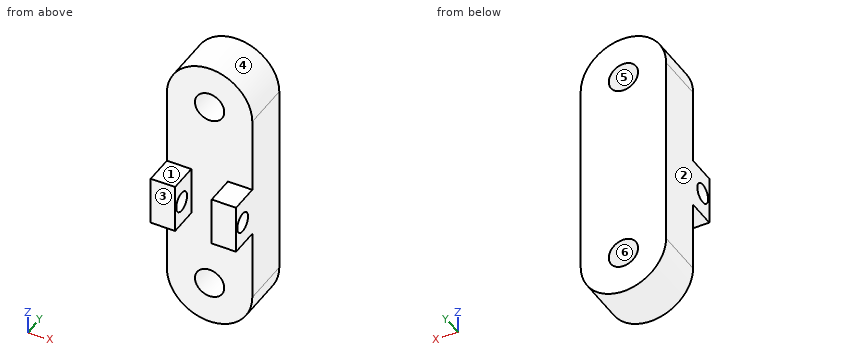
from build123d import *

# Parameters (mm, degrees)
SKETCH1_W             = 5
SKETCH1_H             = 10
BOSS_EXTRUDE1_DEPTH   = 6
BOSS_EXTRUDE1_2_DEPTH = 6
SKETCH2_R             = 2
CUT_EXTRUDE1_DEPTH    = 100
SKETCH4_R             = 3
BOSS_EXTRUDE2_DEPTH   = 10


with BuildPart() as part:
    # Sketch1 → Boss-Extrude1 (new body)
    with BuildSketch(Plane(origin=(0, 0, 0), x_dir=(1, 0, 0), z_dir=(0, 1, 0))):
        with Locations((-15, 5)):
            Rectangle(SKETCH1_W, SKETCH1_H)
    extrude(amount=BOSS_EXTRUDE1_DEPTH)


with BuildPart() as body_2:
    # Sketch1 → Boss-Extrude1 2 (new body)
    with BuildSketch(Plane(origin=(0, 0, 0), x_dir=(1, 0, 0), z_dir=(0, 1, 0))):
        with Locations((-2.5, 5)):
            Rectangle(SKETCH1_W, SKETCH1_H)
    extrude(amount=BOSS_EXTRUDE1_2_DEPTH)


with BuildPart() as cut_extrude1_tool:
    # Sketch2 → Cut-Extrude1 (new body)
    with BuildSketch(Plane(origin=(0, 0, 0), x_dir=(0, 0, -1), z_dir=(1, 0, 0))):
        with Locations((5, 2.43)):
            Circle(SKETCH2_R)
    extrude(amount=-CUT_EXTRUDE1_DEPTH)


with BuildPart() as part_1:
    add(part.part)

    # Cut-Extrude1: cut by cut_extrude1_tool
    add(cut_extrude1_tool.part, mode=Mode.SUBTRACT)



with BuildPart() as body_2_1:
    add(body_2.part)

    # Cut-Extrude1: cut by cut_extrude1_tool
    add(cut_extrude1_tool.part, mode=Mode.SUBTRACT)


with BuildPart() as part_2:
    add(part_1.part)

    add(body_2_1.part)  # Boss-Extrude2 merges body 2
    # Sketch4 → Boss-Extrude2 (add)
    with BuildSketch(Plane(origin=(0, 6, 0), x_dir=(1, 0, 0), z_dir=(0, 1, 0))):
        with BuildLine():
            Line((-17.5, -15.5), (-17.5, 24.5))
            ThreePointArc((-17.5, 24.5), (-8.75, 33.25), (0, 24.5))
            Line((0, 24.5), (0, -15.5))
            ThreePointArc((0, -15.5), (-8.75, -24.25), (-17.5, -15.5))
        make_face()
        with Locations(Location((-8.75, 24.5, 0), (0, 0, 270))):
            Circle(SKETCH4_R, mode=Mode.SUBTRACT)
        with Locations(Location((-8.75, -15.5, 0), (0, 0, 270))):
            Circle(SKETCH4_R, mode=Mode.SUBTRACT)
    extrude(amount=BOSS_EXTRUDE2_DEPTH)


solid = part_2.part
Verification items for the finished model (mm, model axes). Face numbers are marked on the shaded views. A direction names the side the tool comes from. Coordinates: 2 decimals unless noted, no trailing zeros. Order: outer loops, then holes, each group sorted by start corner. A loop starts at its lowest first (then second) coordinate and runs counter-clockwise, first axis right, second up. Notation, with made-up numbers: M 81,38.5 L 119,38.5 A14 ccw 119,48.5 Z; hole C 26.25,70.25 d8. An arc over 180 degrees is marked long. One line per item, written item: value. Start each with the question number.
Item 1: Depth check by flat-ended pin: P1, Ø1, axis at x = -8.5, z = -0.5, coming from the -Y side; P2, Ø3, axis at y = 2.5, z = -4, coming from the -X side; P3, Ø4, axis at x = -3, y = 3, coming from the +Z side; P4, Ø4, axis at x = -16, y = 2.5, coming from the -Z side. Enter the tip coordinate at first touch or a pass-through.
Item 2: Access from +Z, -Z, +X, -X, +Y, -Y to the whole of each face (thin tool, end or side, straight path). Record for the marked faces 1 and 2.
Item 3: Sectioned sample at A-A on y = 2.43. Record the cut outline in (x, z).
Item 4: Thickness scan on probe 1 along Y at (x, z) = (-15.65, -5); probe 2 along X at (y, z) = (5.75, -1.5); probe 3 along Y at (x, z) = (-7.5, 11.5). Record the ranges inside material, lowest first.
Item 5: Sectioned sample at D-D on z = -24. Record the cut outline in (x, y).
Item 6: Mould release check, pull along X, two halves, no side actions. Record for the marked faces 3, 4, 5 and 6: pulls with the +X half, pulls with the -X half, needs draft (parallel to the pull), parting line crosses it, or undercut.
Item 7: Sectioned sample at C-C on x = -8.75. Record the cut outline in (y, z), then the cut area to 3 significant figures.
Item 8: Sectioned sample at B-B on z = -5. Record the cut outline in (x, y).
Calculated:
1. P1: y = 6
1. P2: x = -17.5
1. P3: z = 0
1. P4: z = -10
2. face 1: +Z, +X, -X, -Y
2. face 2: +Z, -Z, -X, +Y, -Y
3. outline: M -17.5,-10 L -12.5,-10 L -12.5,-7 L -17.5,-7 Z; M -17.5,-3 L -12.5,-3 L -12.5,0 L -17.5,0 Z; M -5,-10 L 0,-10 L 0,-7 L -5,-7 Z; M -5,-3 L 0,-3 L 0,0 L -5,0 Z
4. probe 1: 0 to 0.43, 4.43 to 16
4. probe 2: -17.5 to -12.5, -5 to 0
4. probe 3: 6 to 16
5. outline: M -17.5,6 L -11.71,6 L -11.71,16 L -17.5,16 Z; M -5.79,6 L 0,6 L 0,16 L -5.79,16 Z
6. face 3: needs draft
6. face 4: parting line crosses it
6. face 5: undercut
6. face 6: undercut
7. outline: M 6,-33.25 L 16,-33.25 L 16,-27.5 L 6,-27.5 Z; M 6,-21.5 L 16,-21.5 L 16,12.5 L 6,12.5 Z; M 6,18.5 L 16,18.5 L 16,24.25 L 6,24.25 Z
7. area: 455 mm^2
8. outline: M -17.5,0 L -12.5,0 L -12.5,0.43 L -17.5,0.43 Z; M -17.5,4.43 L -12.5,4.43 L -12.5,6 L -5,6 L -5,4.43 L 0,4.43 L 0,16 L -17.5,16 Z; M -5,0 L 0,0 L 0,0.43 L -5,0.43 Z
